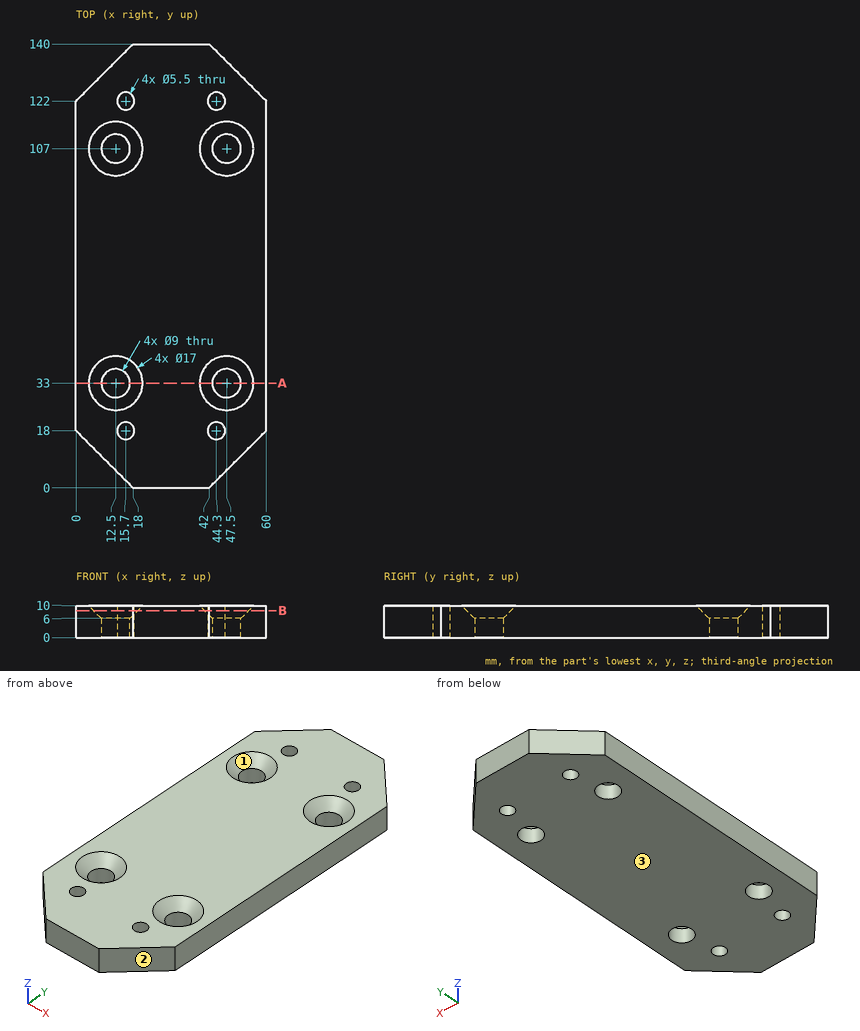
Study the drawing (mm; zero at the part's minimum x, y, z) and answer. Give positions to 0.01 mm unless a question says otherwise; leave off trailing zeros. Loops run counter-clockwise (first coordinate to the right, second up) from the corner with the lowest first, then second, coordinate; pieces in that order, holes last. Notation, with made-up numbers: M -29,-31 L -10,-31 A14 cw -10,-14 Z; hole C -27.75,-26.5 d10. An arc over 180 degrees is marked long. One line per item, written item: value.
1. Section B-B on z = 8.5 is taken. State how many separate pieces and enclosed holes the cut face has, plus the area to 3 significant figures.
Found:
separate pieces: 1
enclosed holes: 8
area: 7,040 mm^2
2. Find the intervals of material crossed by probe 1 along Y at (x, z) = (44.3, 3.5); probe 2 along Y at (x, z) = (12.5, 4.65); probe 3 along X at (y, z) = (123.5, 3), in increasing order.
Found:
probe 1: 2.3 to 15.25, 20.75 to 29.84, 36.16 to 103.84, 110.16 to 119.25, 124.75 to 137.7
probe 2: 5.5 to 28.5, 37.5 to 102.5, 111.5 to 134.5
probe 3: 1.5 to 13.4, 18 to 42, 46.6 to 58.5
3. Section A-A on y = 33 is taken. Determine the outline of the cut face in (x, z).
Found:
outline: M 0,0 L 8,0 L 8,6 L 4,10 L 0,10 Z; M 17,0 L 43,0 L 43,6 L 39,10 L 21,10 L 17,6 Z; M 52,0 L 60,0 L 60,10 L 56,10 L 52,6 Z
4. Each of these flat-tipped pins is pushed along its axis until it touches: P1, Ø1, axis at x = 43.5, y = 59, coming from the -Z side; P2, Ø14.5, axis at x = 47.5, y = 107, coming from the +Z side; P3, Ø1.5, axis at x = 12, z = 8, coming from the +Y side. Where does it stop, or does it pass through?
Found:
P1: z = 0
P2: z = 8.75
P3: y = 134.75
5. For a pull along X with two mould halves and no side action, classify the marked faces 1, 2 and 3 as pulls with the +X half, pulls with the -X half, needs draft (parallel to the pull), parting line crosses it, or undercut.
Found:
face 1: undercut
face 2: pulls with the +X half
face 3: needs draft
